```python
from build123d import *

# Parameters (mm, degrees)
F0_W     = 1219.2
F0_H     = 609.6
F1_DEPTH = 25.4
F2_W     = 1117.6
F2_H     = 508
F2_W_2   = 1066.8
F2_H_2   = 457.2
F3_DEPTH = 76.2
F4_W     = 50.8
F4_H     = 50.8
F4_W_2   = 52.8930136204
F5_DEPTH = 660.4
F6_R     = 25.39999
F7_SIZE  = 25.4


# Not quite as in the source:
# - a fillet or chamfer is up to 0.001 mm smaller than in the source, because OpenCascade refuses the exact size


with BuildPart() as f1:
    # F0 (on Top) → F1 (new body)
    with BuildSketch(Plane.XY):
        Rectangle(F0_W, F0_H)
    extrude(amount=F1_DEPTH)

    # F2 (on face) → F3 (join)
    with BuildSketch(Plane(origin=(0, 0, 0), x_dir=(1, 0, 0), z_dir=(0, 0, -1))):
        Rectangle(F2_W, F2_H)
        Rectangle(F2_W_2, F2_H_2, mode=Mode.SUBTRACT)
    extrude(amount=F3_DEPTH)

    # F4 (on face) → F5 (join)
    with BuildSketch(Plane(origin=(0, 0, 0), x_dir=(1, 0, 0), z_dir=(0, 0, -1))):
        with Locations((-508, 203.2)):
            Rectangle(F4_W, F4_H)
        with Locations((-508, -203.2)):
            Rectangle(F4_W, F4_H)
        with Locations((506.9534931898, -203.2)):
            Rectangle(F4_W_2, F4_H)
        with Locations((508, 203.2)):
            Rectangle(F4_W, F4_H)
    extrude(amount=F5_DEPTH)

    # F6 (radius 25.4 in the source; OpenCascade refuses exactly that, so slightly less here)
    f6_edges = [f1.edges().sort_by_distance(p)[0] for p in [
        (0, 304.8, 0),
        (-609.6, 0, 0),
        (609.6, 0, 0),
        (0, -304.8, 0),
    ]]
    fillet(f6_edges, radius=F6_R)

    # F7
    f7_edges = [f1.edges().sort_by_distance(p)[0] for p in [
        (-533.4, -228.6, -368.3),
        (-533.4, 228.6, -368.3),
        (533.4, 228.6, -368.3),
        (533.4, -228.6, -368.3),
    ]]
    chamfer(f7_edges, length=F7_SIZE)


solid = f1.part
```
The model under review builds one solid part; all positions refer to its coordinate system, in mm. A direction names the side the tool comes from. Coordinates: 2 decimals unless noted, no trailing zeros. Write each loop counter-clockwise with the first axis right and the second up, starting at its lowest first coordinate (ties: lowest second). Pieces come first, ordered by that corner, then holes. Notation, with made-up numbers: (30, 23.5) - (45, 23.5) arc R16 cw to (45, 34.5) - close; hole circle Ø6 at (73, 9.5). An arc over 180 degrees is marked (long way). Write item = value, one per line.
(1) Consider section C-C, the plane z = -487.5. Give the boundary of the cut face in (x, y).
Result sheet:
outline = (-533.4, -203.2) - (-508, -228.6) - (-482.6, -228.6) - (-482.6, -177.8) - (-533.4, -177.8) - close; (-533.4, 177.8) - (-482.6, 177.8) - (-482.6, 228.6) - (-508, 228.6) - (-533.4, 203.2) - close; (480.51, 177.8) - (533.4, 177.8) - (533.4, 203.2) - (508, 228.6) - (480.51, 228.6) - close; (482.6, -228.6) - (508, -228.6) - (533.4, -203.2) - (533.4, -177.8) - (482.6, -177.8) - close
(2) For line 1 (X direction, y = -175.5, z = -46.5); line 2 (X direction, y = 178.5, z = -176); line 3 (Y direction, x = -140.5, z = -19), list the stretches that pass through material, from the lowest coordinate up. Write a range as [from, to].
Result sheet:
line_1 = [-558.8, -533.4], [533.4, 558.8]
line_2 = [-533.4, -482.6], [480.51, 533.4]
line_3 = [-254, -228.6], [228.6, 254]
(3) Mouldability with a two-part tool opening along Y and no side actions: class faces 6 (the face through (8.53, -297.16, 7.24)), 7 (the face through (533.4, -190, -364)), 8 (the face through (533.4, 2, -38)), 9 (the face through (520.9, 215.7, -364.2)) as pulls with the +Y half, pulls with the -Y half, needs draft (parallel to the pull), parting line crosses it, or undercut.
Result sheet:
face_6 = pulls with the -Y half
face_7 = needs draft
face_8 = undercut
face_9 = pulls with the +Y half
(4) Machinability: for faces 1 (the face through (-520.9, 215.7, -364.2)), 2 (the face through (-8, 254, -38)), 3 (the face through (-8, 228.6, -38)), 4 (the face through (-533.4, 191, -364)), 5 (the face through (520.5, -216.1, -364.2)), which of the approach directions +Z, -Z, +X, -X, +Y, -Y give a long, thin tool a straight path to every point of the face, cutting with its end or side? Answer none if there is none.
Result sheet:
face_1 = -Z, -X, +Y
face_2 = -Z, +X, -X, +Y
face_3 = -Z
face_4 = -Z, -X, +Y, -Y
face_5 = -Z, +X, -Y
(5) Consider section A-A, the plane z = -21. Give the boundary of the cut face in (x, y), then the cut area to 3 significant figures.
Result sheet:
outline = (-558.8, -254) - (558.8, -254) - (558.8, 254) - (-558.8, 254) - close; hole (-533.4, -177.8) - (-482.6, -177.8) - (-482.6, -228.6) - (482.6, -228.6) - (482.6, -177.8) - (533.4, -177.8) - (533.4, 177.8) - (480.51, 177.8) - (480.51, 228.6) - (-482.6, 228.6) - (-482.6, 177.8) - (-533.4, 177.8) - close
area = 90,400 mm^2
(6) For P1, Ø12.5, axis at y = 192, z = -414.5, coming from the -X side; P2, Ø1, axis at x = -458, y = -239.5, coming from the -Z side; P3, Ø8, axis at x = -463, y = -44.5, coming from the -Z side, all flat-tipped, find the tip position at first contact; note any pin that passes through.
Result sheet:
P1 = -533.4
P2 = -76.2
P3 = 0
